```python
from build123d import *

# Parameters (mm, degrees)
PAD_DEPTH       = 20
FILLET_R        = 0.5
FILLET001_R     = 0.5
FILLET002_R     = 0.4
FILLET003_R     = 0.4
SKETCH002_W     = 6.171573
SKETCH002_H     = 16.569204
POCKET_DEPTH    = 23
SKETCH003_W     = 6.204978
SKETCH003_H     = 16.552317
SKETCH003_H_2   = 16.575784
POCKET001_DEPTH = 23
FILLET004_R     = 0.4
FILLET005_R     = 0.4
FILLET006_R     = 0.4
FILLET007_R     = 0.4
FILLET008_R     = 0.4
FILLET009_R     = 0.4
FILLET010_R     = 0.4
FILLET011_R     = 0.4


with BuildPart() as part:
    # Sketch → Pad (new body)
    with BuildSketch(Plane.YZ):
        Polygon((-9.999999, 0), (10.000001, 0), (10.000001, 1.2), (1.4, 1.2), (1.4, 3.6), (0.2, 3.6), (0.2, 1.2), (-0.2, 1.2), (-0.2, 3.6), (-1.4, 3.6), (-1.4, 1.2), (-10.000001, 1.2), align=None)
    extrude(amount=PAD_DEPTH)

    # Fillet
    fillet_edges = [part.edges().sort_by_distance(p)[0] for p in [
        (10, -10.000001, 1.2),
    ]]
    fillet(fillet_edges, radius=FILLET_R)

    # Fillet001
    fillet001_edges = [part.edges().sort_by_distance(p)[0] for p in [
        (10, 10.000001, 1.2),
    ]]
    fillet(fillet001_edges, radius=FILLET001_R)

    # Fillet002
    fillet002_edges = [part.edges().sort_by_distance(p)[0] for p in [
        (10, -1.4, 1.2),
    ]]
    fillet(fillet002_edges, radius=FILLET002_R)

    # Fillet003
    fillet003_edges = [part.edges().sort_by_distance(p)[0] for p in [
        (10, 1.4, 1.2),
    ]]
    fillet(fillet003_edges, radius=FILLET003_R)

    # Sketch002 → Pocket (cut)
    with BuildSketch(Plane(origin=(0, 0, 1.2), x_dir=(0, -1, 0), z_dir=(0, 0, 1))):
        with Locations((-5.631366, 10)):
            Rectangle(SKETCH002_W, SKETCH002_H)
    extrude(amount=-POCKET_DEPTH, mode=Mode.SUBTRACT)

    # Sketch003 → Pocket001 (cut)
    with BuildSketch(Plane(origin=(0, 0, 1.2), x_dir=(0, -1, 0), z_dir=(0, 0, 1))):
        with Locations((5.641938, 10.014704)):
            Rectangle(SKETCH003_W, SKETCH003_H)
        with Locations((-5.641938, 10.002971)):
            Rectangle(SKETCH003_W, SKETCH003_H_2)
    extrude(amount=-POCKET001_DEPTH, mode=Mode.SUBTRACT)

    # Fillet004
    fillet004_edges = [part.edges().sort_by_distance(p)[0] for p in [
        (1.738546, -5.641938, 1.2),
        (10.014704, -2.539449, 1.2),
        (10.014705, -8.744427, 1.2),
        (18.290863, -5.641938, 1.2),
    ]]
    fillet(fillet004_edges, radius=FILLET004_R)

    # Fillet005
    fillet005_edges = [part.edges().sort_by_distance(p)[0] for p in [
        (10.002971, 8.744427, 1.2),
        (1.715079, 5.641938, 1.2),
        (10.002971, 2.539449, 1.2),
        (18.290863, 5.641938, 1.2),
    ]]
    fillet(fillet005_edges, radius=FILLET005_R)

    # Fillet006
    fillet006_edges = [part.edges().sort_by_distance(p)[0] for p in [
        (10, -1.4, 3.6),
    ]]
    fillet(fillet006_edges, radius=FILLET006_R)

    # Fillet007
    fillet007_edges = [part.edges().sort_by_distance(p)[0] for p in [
        (10, 1.4, 3.6),
    ]]
    fillet(fillet007_edges, radius=FILLET007_R)

    # Fillet008
    fillet008_edges = [part.edges().sort_by_distance(p)[0] for p in [
        (20, -0.6, 3.6),
    ]]
    fillet(fillet008_edges, radius=FILLET008_R)

    # Fillet009
    fillet009_edges = [part.edges().sort_by_distance(p)[0] for p in [
        (20, 0.6, 3.6),
    ]]
    fillet(fillet009_edges, radius=FILLET009_R)

    # Fillet010
    fillet010_edges = [part.edges().sort_by_distance(p)[0] for p in [
        (0, -0.6, 3.6),
    ]]
    fillet(fillet010_edges, radius=FILLET010_R)

    # Fillet011
    fillet011_edges = [part.edges().sort_by_distance(p)[0] for p in [
        (0, 0.6, 3.6),
    ]]
    fillet(fillet011_edges, radius=FILLET011_R)


solid = part.part
```
Can you work these out from the model? Positions are in its coordinate system, mm. A direction names the side the tool comes from. Coordinates: 2 decimals unless noted, no trailing zeros. Order: outer loops, then holes, each group sorted by start corner. A loop starts at its lowest first (then second) coordinate and runs counter-clockwise, first axis right, second up.
1. If we section it at B-B (y = -8.25): Please give me the cut outline in (x, z).
2. If we section it at D-D (y = 8.5): Please give me the cut outline in (x, z).
3. For faces 4 (the face through (20, 0, 1)), 5 (the face through (9.96, 1.96, 1.2)), 6 (the face through (10, -9.3, 1.2)), 7 (the face through (10, -0.2, 2)), 8 (the face through (10, 0, 0)), which set-ups out of +Z, -Z, +X, -X, +Y, -Y let a thin tool reach every point of the face, with its end or its side?
4. I'm going to push flat-ended pins straight in: pin 1 (0.5 mm diameter, centred on x = 8.5, z = 2.5, fed in from -Y); pin 2 (1.5 mm diameter, centred on x = 4, y = -3, fed in from -Z); pin 3 (8.5 mm diameter, centred on x = 5.5, y = -7, fed in from +Z); pin 4 (1.9 mm diameter, centred on x = 6, z = 2, fed in from +Y). Where does each tip first touch, or does it pass through?
5. Thinking about a two-plate mould opening in Y: for faces 1 (the face through (10, 0.2, 2)), 2 (the face through (10, -1.4, 2)), 3 (the face through (0, 0, 1)), which applies, +Y half, -Y half, draft (parallel to the pull), parting line (faces both ways), or undercut?
6. If we section it at A-A (x = 3.75): Give the number of separate pieces and of enclosed holes in the cut face, then the cut area to 3 significant figures.
7. I need wall thicknesses on line 1 (Y direction, x = 2.25, z = 0.55); line 2 (Y direction, x = 10, z = 1.9); line 3 (X direction, y = -2.75, z = 0.7). Which ranges of each line are inside material? Lowest first, please.
Entries:
1. outline: (0, 0) - (1.74, 0) - (1.74, 0.8) arc R0.4 ccw to (1.34, 1.2) - (0.4, 1.2) arc R0.4 ccw to (0, 0.8) - close; (18.29, 0) - (20, 0) - (20, 0.8) arc R0.4 ccw to (19.6, 1.2) - (18.69, 1.2) arc R0.4 ccw to (18.29, 0.8) - close
2. outline: (0, 0) - (1.72, 0) - (1.72, 0.8) arc R0.4 ccw to (1.32, 1.2) - (0.4, 1.2) arc R0.4 ccw to (0, 0.8) - close; (18.29, 0) - (20, 0) - (20, 0.8) arc R0.4 ccw to (19.6, 1.2) - (18.69, 1.2) arc R0.4 ccw to (18.29, 0.8) - close
3. face 4: +Z, -Z, +X, +Y, -Y
3. face 5: +Z, +X, -X, +Y
3. face 6: +Z, +X, -X, -Y
3. face 7: +Z, +X, -X
3. face 8: -Z, +X, -X, +Y, -Y
4. pin 1: stops at y = -1.4
4. pin 2: stops at z = 0
4. pin 3: stops at z = 1.2
4. pin 4: stops at y = 9.86
5. face 1: undercut
5. face 2: -Y half
5. face 3: draft
6. separate pieces: 3
6. enclosed holes: 0
6. area: 14.6 mm2
7. line 1: y = -10 to -8.74, -2.54 to 2.54, 8.74 to 10
7. line 2: y = -1.4 to -0.2, 0.2 to 1.4
7. line 3: x = 0 to 1.74, 18.29 to 20
